For this review, take the finished solid that the model builds, in its own axes (mm). A direction names the side the tool comes from. Coordinates: 2 decimals unless noted, no trailing zeros. Write each loop counter-clockwise with the first axis right and the second up, starting at its lowest first coordinate (ties: lowest second). Pieces come first, ordered by that corner, then holes.
1) For faces 4 (the face through (12.71, -17.8, 11.39)), 5 (the face through (-0.75, 16, 11)), list the 3-axis set-ups (+Z, -Z, +X, -X, +Y, -Y) from which the entire face can be reached by the end or side of a thin tool; tool diameter is ignored.
2) We need section D-D on y = -20. Write out the cut boundary in (x, z).
3) We need section B-B on y = 0. Write out the cut boundary in (x, z).
4) Insertion check: P1, Ø1.1, axis at x = -16, y = 4.5, coming from the +Z side; P2, Ø5, axis at x = 22, z = 15.5, coming from the +Y side; P3, Ø4, axis at y = -10.5, z = 23, coming from the -X side. Each pin has a flat end and moves straight along its axis. Give the tip position at first contact, or say it passes through.
5) We need section C-C on x = 14. Write out the cut boundary in (y, z).
6) We need section A-A on x = 0. Write out the cut boundary in (y, z).
7) Mouldability with a two-part tool opening along X and no side actions: class faces 1 (the face through (20.856, 6.589, 11.387)), 2 (the face through (-9, -13, 19)), 3 (the face through (-20.746, 6.929, 11.387)) as pulls with the +X half, pulls with the -X half, needs draft (parallel to the pull), parting line crosses it, or undercut.
8) To check wall thickness, follow line 1 along Y through (x, z) = (0, 18.75); line 2 along Y through (x, z) = (0, 7); line 3 along X through (y, z) = (0, 21.5). State the ranges of each line that lie inside material, in increasing order.
from build123d import *

# Parameters (mm, degrees)
BOSS_EXTRU_1_DEPTH           = 20
COQUE1_T                     = -2.6
BOSS_EXTRU_2_REACH           = 51.719
BOSS_EXTRU_2_END_RADIUS      = 78.3
ESQUISSE4_R                  = 12.5
NERVURE1_REACH               = 45.628
ESQUISSE6_WALLS_W            = 1.5
ESQUISSE6_WALLS_H            = 96.027794688
R_P_TITION_CIRCULAIRE1_COUNT = 5


with BuildPart() as part:
    # Esquisse1 → Boss.-Extru.1 (new body)
    with BuildSketch(Plane.XY):
        with BuildLine():
            ThreePointArc((-12.14837206, 25.22730775), (-16.457987064, 22.652475842), (-20.238542003, 19.349455227))
            ThreePointArc((-20.238542003, 19.349455227), (-20.800515992, 6.758497338), (-27.746648844, -3.758121593))
            ThreePointArc((-27.746648844, -3.758121593), (-26.629582456, -8.652475842), (-24.656478901, -13.268686756))
            ThreePointArc((-24.656478901, -13.268686756), (-12.855425866, -17.693975742), (-5, -27.549954628))
            ThreePointArc((-5, -27.549954628), (0, -28), (5, -27.549954628))
            ThreePointArc((5, -27.549954628), (12.855425866, -17.693975742), (24.656478901, -13.268686756))
            ThreePointArc((24.656478901, -13.268686756), (26.629582456, -8.652475842), (27.746648844, -3.758121593))
            ThreePointArc((27.746648844, -3.758121593), (20.800515992, 6.758497338), (20.238542003, 19.349455227))
            ThreePointArc((20.238542003, 19.349455227), (16.457987064, 22.652475842), (12.14837206, 25.22730775))
            ThreePointArc((12.14837206, 25.22730775), (0, 21.87095681), (-12.14837206, 25.22730775))
        make_face()
    extrude(amount=BOSS_EXTRU_1_DEPTH)

    # Esquisse3 → Enlèvement de matière-Révolution3 (revolve, cut)
    with BuildSketch(Plane(origin=(0, 0, 0), x_dir=(0, 0, -1), z_dir=(1, 0, 0)), mode=Mode.PRIVATE) as enl_vement_de_mati_re_r_volution3_sk:
        with BuildLine():
            Line((-5, -28), (3.997916613, -28))
            Line((3.997916613, -28), (3.997916613, 0))
            Line((3.997916613, 0), (0, 0))
            ThreePointArc((0, 0), (-1.259809141, -14.221462653), (-5, -28))
        make_face()
    revolve(enl_vement_de_mati_re_r_volution3_sk.sketch.rotate(Axis((0, 0, 0), (0, 0, 1)), 180), axis=Axis((0, 0, 0), (0, 0, 1)), mode=Mode.SUBTRACT)

    # Coque1
    coque1_openings = [part.faces().sort_by_distance(p)[0] for p in [
        (0, 0, 20),
    ]]
    offset(amount=COQUE1_T, openings=coque1_openings)

    # Boss.-Extru.2: up to this sphere (the profile starts inside it)
    boss_extru_2_end = Location((0, 0, 80.9)) * Sphere(BOSS_EXTRU_2_END_RADIUS, mode=Mode.PRIVATE)
    # Esquisse4 → Boss.-Extru.2 (add, up to the surface)
    with BuildSketch(Plane.XY.offset(30.3), mode=Mode.PRIVATE) as boss_extru_2_sk1:
        Circle(ESQUISSE4_R)
    boss_extru_2_tool1 = extrude(boss_extru_2_sk1.sketch, amount=-BOSS_EXTRU_2_REACH, mode=Mode.PRIVATE) & boss_extru_2_end
    add(boss_extru_2_tool1.solids().sort_by_distance((0, 0, 30.3))[0])

    # Esquisse5 → Enlèvement de matière-Révolution4 (revolve, cut)
    with BuildSketch(Plane(origin=(0, 0, 0), x_dir=(1, 0, 0), z_dir=(0, 1, 0)), mode=Mode.PRIVATE) as enl_vement_de_mati_re_r_volution4_sk:
        Polygon((0, -30.3), (8, -30.3), (8, -14.3), (7, -14.3), (7, 4.215006275), (0, 4.215006275), align=None)
    revolve(enl_vement_de_mati_re_r_volution4_sk.sketch.rotate(Axis((0, 0, 0), (0, 0, 1)), 115.713439389), axis=Axis((0, 0, 0), (0, 0, 1)), mode=Mode.SUBTRACT)

    # Esquisse6 walls → Nervure1 (add, up to next)
    with BuildSketch(Plane.XY.offset(19), mode=Mode.PRIVATE) as nervure1_sk1:
        with Locations((0, 15.885478405)):
            Rectangle(ESQUISSE6_WALLS_W, ESQUISSE6_WALLS_H)
    nervure1_tool1 = extrude(nervure1_sk1.sketch, amount=-NERVURE1_REACH, mode=Mode.PRIVATE) - part.part
    nervure1 = nervure1_tool1.solids().sort_by_distance((0, 15.885478405, 19))[0]
    add(nervure1)

    # Répétition circulaire1: Nervure1 ×5 about axis
    r_p_tition_circulaire1_axis = Axis((0, 0, 0), (0, 0, -1))
    for i in range(1, R_P_TITION_CIRCULAIRE1_COUNT):
        add(nervure1.rotate(r_p_tition_circulaire1_axis, i * 360 / R_P_TITION_CIRCULAIRE1_COUNT))


solid = part.part
Result:
1. face 4: +Z, -Z, +X, -Y
1. face 5: +Z
2. outline: (-10.14, 3.17) arc R78.39 ccw to (10.14, 3.17) - (10.14, 20) - (6.61, 20) - (6.61, 5.49) arc R75.7 cw to (-6.61, 5.49) - (-6.61, 20) - (-10.14, 20) - close
3. outline: (-24.28, 3.73) arc R80.9 ccw to (-7, 0.3) - (-7, 14.3) - (-8, 14.3) - (-8, 30.3) - (-12.5, 30.3) - (-12.5, 3.6) arc R78.3 cw to (-21.13, 5.5) - (-21.13, 20) - (-24.28, 20) - close; (7, 0.3) arc R80.9 ccw to (24.28, 3.73) - (24.28, 20) - (21.13, 20) - (21.13, 5.5) arc R78.3 cw to (12.5, 3.6) - (12.5, 30.3) - (8, 30.3) - (8, 14.3) - (7, 14.3) - close
4. P1: stops at z = 19
4. P2: stops at y = 20.09
4. P3: stops at x = -9.17
5. outline: (-16.91, 3.04) arc R79.68 ccw to (24.25, 5) - (24.25, 20) - (21.19, 20) - (21.19, 6.83) arc R77.04 cw to (5.34, 4.05) - (5.34, 19) - (3.76, 19) - (3.76, 3.95) arc R77.04 cw to (-13.89, 5.12) - (-13.89, 20) - (-16.91, 20) - close
6. outline: (-28, 5) arc R80.9 ccw to (-7, 0.3) - (-7, 14.3) - (-8, 14.3) - (-8, 30.3) - (-12.5, 30.3) - (-12.5, 3.6) arc R78.3 cw to (-25.4, 6.83) - (-25.4, 20) - (-28, 20) - close; (7, 0.3) arc R80.9 ccw to (21.87, 3.01) - (21.87, 20) - (19.27, 20) - (19.27, 19) - (12.5, 19) - (12.5, 30.3) - (8, 30.3) - (8, 14.3) - (7, 14.3) - close
7. face 1: pulls with the +X half
7. face 2: undercut
7. face 3: pulls with the -X half
8. line 1: y = -28 to -25.4, -12.5 to -8, 8 to 21.87
8. line 2: y = -28 to -25.4, -12.5 to -7, 7 to 21.87
8. line 3: x = -12.5 to -8, 8 to 12.5
